```python
from build123d import *

# Parameters (mm, degrees)
F0_R     = 14
F1_DEPTH = 70


with BuildPart() as f1:
    # F0 (on Front) → F1 (new body)
    with BuildSketch(Plane.XZ):
        with BuildLine():
            Line((-119, -46.5), (-119, -56))
            Line((-119, -56), (0, -56))
            Line((0, -56), (0, -14))
            ThreePointArc((0, -14), (-9.899495, -9.899495), (-14, 0))
            ThreePointArc((-14, 0), (-9.899495, 9.899495), (0, 14))
            Line((0, 14), (0, 56))
            Line((0, 56), (-1.5, 56))
            ThreePointArc((-1.5, 56), (-4, 53.5), (-6.5, 56))
            Line((-6.5, 56), (-9.5, 56))
            ThreePointArc((-9.5, 56), (-12, 53.5), (-14.5, 56))
            Line((-14.5, 56), (-17.5, 56))
            ThreePointArc((-17.5, 56), (-20, 53.5), (-22.5, 56))
            Line((-22.5, 56), (-25.5, 56))
            ThreePointArc((-25.5, 56), (-28, 53.5), (-30.5, 56))
            Line((-30.5, 56), (-33.5, 56))
            ThreePointArc((-33.5, 56), (-36, 53.5), (-38.5, 56))
            Line((-38.5, 56), (-41.5, 56))
            ThreePointArc((-41.5, 56), (-44, 53.5), (-46.5, 56))
            Line((-46.5, 56), (-49.5, 56))
            ThreePointArc((-49.5, 56), (-52, 53.5), (-54.5, 56))
            Line((-54.5, 56), (-57.5, 56))
            ThreePointArc((-57.5, 56), (-60, 53.5), (-62.5, 56))
            Line((-62.5, 56), (-65.5, 56))
            ThreePointArc((-65.5, 56), (-68, 53.5), (-70.5, 56))
            Line((-70.5, 56), (-73.5, 56))
            ThreePointArc((-73.5, 56), (-76, 53.5), (-78.5, 56))
            Line((-78.5, 56), (-81.5, 56))
            ThreePointArc((-81.5, 56), (-84, 53.5), (-86.5, 56))
            Line((-86.5, 56), (-89.5, 56))
            ThreePointArc((-89.5, 56), (-92, 53.5), (-94.5, 56))
            Line((-94.5, 56), (-97.5, 56))
            ThreePointArc((-97.5, 56), (-100, 53.5), (-102.5, 56))
            Line((-102.5, 56), (-119, 56))
            Line((-119, 56), (-119, 46.5))
            ThreePointArc((-119, 46.5), (-116.5, 44), (-119, 41.5))
            Line((-119, 41.5), (-119, 38.5))
            ThreePointArc((-119, 38.5), (-116.5, 36), (-119, 33.5))
            Line((-119, 33.5), (-119, 30.5))
            ThreePointArc((-119, 30.5), (-116.5, 28), (-119, 25.5))
            Line((-119, 25.5), (-119, 22.5))
            ThreePointArc((-119, 22.5), (-116.5, 20), (-119, 17.5))
            Line((-119, 17.5), (-119, 14.5))
            ThreePointArc((-119, 14.5), (-116.5, 12), (-119, 9.5))
            Line((-119, 9.5), (-119, 6.5))
            ThreePointArc((-119, 6.5), (-116.5, 4), (-119, 1.5))
            Line((-119, 1.5), (-119, -1.5))
            ThreePointArc((-119, -1.5), (-116.5, -4), (-119, -6.5))
            Line((-119, -6.5), (-119, -9.5))
            ThreePointArc((-119, -9.5), (-116.5, -12), (-119, -14.5))
            Line((-119, -14.5), (-119, -17.5))
            ThreePointArc((-119, -17.5), (-116.5, -20), (-119, -22.5))
            Line((-119, -22.5), (-119, -25.5))
            ThreePointArc((-119, -25.5), (-116.5, -28), (-119, -30.5))
            Line((-119, -30.5), (-119, -33.5))
            ThreePointArc((-119, -33.5), (-116.5, -36), (-119, -38.5))
            Line((-119, -38.5), (-119, -41.5))
            ThreePointArc((-119, -41.5), (-116.5, -44), (-119, -46.5))
        make_face()
        with Locations((-95, -32)):
            Circle(F0_R, mode=Mode.SUBTRACT)
        with Locations((-57, -32)):
            Circle(F0_R, mode=Mode.SUBTRACT)
        with Locations((-19, -32)):
            Circle(F0_R, mode=Mode.SUBTRACT)
        with BuildLine():
            Line((-109, -13.076697), (-109, 13.076697))
            ThreePointArc((-109, 13.076697), (-100, 0), (-109, -13.076697))
        make_face(mode=Mode.SUBTRACT)
        with Locations((-76, 0)):
            Circle(F0_R, mode=Mode.SUBTRACT)
        with Locations((-95, 32)):
            Circle(F0_R, mode=Mode.SUBTRACT)
        with Locations((-38, 0)):
            Circle(F0_R, mode=Mode.SUBTRACT)
        with Locations((-57, 32)):
            Circle(F0_R, mode=Mode.SUBTRACT)
        with Locations((-19, 32)):
            Circle(F0_R, mode=Mode.SUBTRACT)
    extrude(amount=-F1_DEPTH)


solid = f1.part
```
The model under review builds one solid part; all positions refer to its coordinate system, in mm. Round coordinates to 2 decimals unless told otherwise and drop trailing zeros. Loops run counter-clockwise (first coordinate to the right, second up) from the corner with the lowest first, then second, coordinate; pieces in that order, holes last. Notation, with made-up numbers: M 51.5,16.5 L 62.5,16.5 A6 cw 62.5,26.5 Z; hole C -17,5.5 d9. An arc over 180 degrees is marked long. Answer as a JSON object with one key per item and string values.
(1) Take a section at A-A on z = -32. Give the boundary of the cut face in (x, y), and give its area (3 significant figures).
Resolved:
{"outline": "M -119,0 L -109,0 L -109,70 L -119,70 Z; M -81,0 L -71,0 L -71,70 L -81,70 Z; M -43,0 L -33,0 L -33,70 L -43,70 Z; M -5,0 L 0,0 L 0,70 L -5,70 Z", "area": "2,450 mm²"}
(2) Clearance check with a flat-ended pin moving along its axis: P1, Ø17, axis at x = -19, z = 32, coming from the -Y side. State where the tip first meets the part, or that it passes through.
Resolved:
{"P1": "through"}
(3) Take a section at B-B on x = -67. Give the boundary of the cut face in (y, z), and give its area (3 significant figures).
Resolved:
{"outline": "M 0,-56 L 70,-56 L 70,-41.8 L 0,-41.8 Z; M 0,-22.2 L 70,-22.2 L 70,-10.72 L 0,-10.72 Z; M 0,10.72 L 70,10.72 L 70,22.2 L 0,22.2 Z; M 0,41.8 L 70,41.8 L 70,53.71 L 0,53.71 Z", "area": "3,430 mm²"}
(4) To check wall thickness, follow line 1 along Z through (x, y) = (-95, 43); line 2 along Z through (x, y) = (-76, 44); line 3 along Z through (x, y) = (-90.5, 44.5). State the ranges of each line that lie inside material, in increasing order.
Resolved:
{"line 1": "-56 to -46, -18 to 18, 46 to 56", "line 2": "-56 to -14, 14 to 53.5", "line 3": "-56 to -45.26, -18.74 to 18.74, 45.26 to 54"}
(5) Take a section at D-D on y = 52. Count the separate pieces of the cut face and the enclosed holes in it, and give its area (3 significant figures).
Resolved:
{"separate pieces": "1", "enclosed holes": "9", "area": "7,680 mm²"}
(6) Take a section at C-C on x = -96. Give the boundary of the cut face in (y, z).
Resolved:
{"outline": "M 0,-56 L 70,-56 L 70,-45.96 L 0,-45.96 Z; M 0,-18.04 L 70,-18.04 L 70,18.04 L 0,18.04 Z; M 0,45.96 L 70,45.96 L 70,56 L 0,56 Z"}
(7) Draft analysis for pull direction X (two halves, no side actions). For faces 1 (the cylindrical face through (-27.9, 34.5, 53.5)), 2 (the flat face through (-119, 35, -51)), 3 (the flat face through (-16, 35, 56)), state which applies: released by +X, released by -X, zero draft, split by the parting line, or undercut.
Resolved:
{"face 1": "undercut", "face 2": "released by -X", "face 3": "zero draft"}
